Can you work these out from the model? Positions are in its coordinate system, mm. Face numbers are marked on the shaded views. A direction names the side the tool comes from. Give positions to 0.01 mm unless a question says otherwise; leave off trailing zeros. Order: outer loops, then holes, each group sorted by start corner. A loop starts at its lowest first (then second) coordinate and runs counter-clockwise, first axis right, second up. Notation, with made-up numbers: (-4, 80.5) - (47, 80.5) arc R7 ccw to (47, 88.5) - close; hole circle Ø4 at (15, -8). An arc over 180 degrees is marked (long way). Use one line per item in the form item = value. Start each with the question number.
1) For pin 1 (6 mm diameter, centred on x = -25, z = -1.5, fed in from -Y); pin 2 (3 mm diameter, centred on x = -4, y = 9, fed in from +Z); pin 3 (0.8 mm diameter, centred on x = -11, y = 8, fed in from +Z); pin 4 (8 mm diameter, centred on x = -32, y = 8.5, fed in from -Z), each with a flat end and sliding along its axis, tell me the tip position at first contact or that it passes through.
2) Please list where these lines run through material, in increasing order: probe 1 along Y at (x, z) = (-31, -3); probe 2 along X at (y, z) = (-2.75, -16); probe 3 along Y at (x, z) = (20, -6.75).
3) We'd pull the mould along X, two halves only. Please class the marked faces 1, 2 and 3: released by +X, released by -X, zero draft, split by the parting line, or undercut.
4) Suppose I cut it at D-D, the plane x = 27. Write out the boundary of the cut face in (y, z), and give its area (3 significant figures).
5) Suppose I cut it at B-B, the plane z = -1.25. Write out the boundary of the cut face in (x, y) (3 decimals), and give its area (3 significant figures).
6) Suppose I cut it at C-C, the plane x = 7.5. Write out the boundary of the cut face in (y, z).
7) Suppose I cut it at A-A, the plane y = -1.5. Write out the boundary of the cut face in (x, z) (1 decimal).
8) Which directions (+Z, -Z, +X, -X, +Y, -Y) give clear straight access to the entire face, cutting with the end or side of a thin tool? Please do the marked faces 4, 5 and 6.
Autodesk Inventor part; units mm, degrees
ref_plane "YZ Plane" through (0, 0, 0) normal (1, 0, 0) x (0, 1, 0)
ref_plane "XZ Plane" through (0, 0, 0) normal (0, 1, 0) x (-1, 0, 0)
ref_plane "XY Plane" through (0, 0, 0) normal (0, 0, 1) x (1, 0, 0)
sketch "Sketch1" plane through (0, 0, 0) normal (0, 0, 1) x (1, 0, 0)
  line L0 (0, 12.3444) -> (0, -2.0574)
  line L1 (-35.56, 0) -> (35.56, 0)
  line L2 (-35.56, 0) -> (35.56, 0)
  line L3 (0, -2.0574) -> (0, 12.3444)
  line L4 (-12.319, 8.2169) -> (15.113, 8.2169)
  line L5 (-10.2108, 8.2169) -> (13.0048, 8.2169)
  circle A0 centre (-11.2649, 8.2169) radius 1.0541
  circle A1 centre (14.0589, 8.2169) radius 1.0541
  line L6 (-25.4, 10.287) -> (-25.4, 0)
  line L7 (-25.4, 0) -> (25.4, 0)
  line L8 (-25.4, 10.287) -> (25.4, 10.287)
  line L9 (25.4, 10.287) -> (25.4, 0)
  line L10 (25.4, 10.287) -> (14.0589, 10.287)
  line L11 (14.0589, 10.287) -> (14.0589, 7.1628)
  line L12 (14.0589, 9.271) -> (14.0589, 10.287)
  line L13 (14.0589, 8.2169) -> (15.113, 8.2169)
  circle A2 centre (-11.2649, 8.2169) radius 0.8001
  circle A3 centre (14.0589, 8.2169) radius 0.8001
  point P0 (0, 0)
  dimension "d0" = 27.432
  dimension "d1" = 23.2156
  dimension "d2" = 2.1082
  dimension "d3" = 10.287
  dimension "d4" = 50.8
  dimension "d5" = 11.3411
  dimension "d6" = 1.016
  dimension "d7" = 11.3411
  dimension "d8" = 0.254
  dimension "d9" = 0.254
extrude "Extrusion1" add sketch "Sketch1" against normal blind 5.08 contours L8 L11 A1 L4 L0 | L0 L1 L6 L8 | L4 A1 L11 L8 L9 L1 L0
extrude "Extrusion2" add sketch "Sketch1" against normal blind 5.08 contours A0 L4 A2 | L4 A2 A0 | A1 L11 A3 L4 | L4 A3 L11 A1 | A1 L4 A3 L11 | A2 L4 | L4 A2 | A3 L11 L4 | L4 L11 A3 | L11 A3 L4 A1 | A3 L4 L11 | L4 A3 L11
extrude "Extrusion3" add sketch "Sketch1" along normal blind 2.032 contours A2 L4 | L4 A2 | A3 L11 L4 | L4 L11 A3 | A3 L4 L11 | L4 A3 L11
sketch "Sketch2" plane through (-25.4, 0, 0) normal (0, -1, 0) x (1, 0, 0)
  line L0 (50.8, 0) -> (50.8, -5.08)
  line L1 (0, 0) -> (50.8, 0)
  line L2 (0, 0) -> (0, -5.08)
  line L3 (38.1, -5.08) -> (12.7, -5.08)
  line L4 (12.7, -17.78) -> (38.1, -17.78)
  arc A0 (38.1, -12.7) -> (38.1, -10.16) centre (38.1, -11.43) ccw
  arc A1 (12.7, -10.16) -> (12.7, -12.7) centre (12.7, -11.43) ccw
  line L5 (38.1, -17.78) -> (38.1, -12.7)
  line L6 (38.1, -10.16) -> (38.1, -5.08)
  line L7 (12.7, -5.08) -> (12.7, -10.16)
  line L8 (12.7, -12.7) -> (12.7, -17.78)
  line L9 (50.8, 0) -> (0, 0)
  line L10 (25.4, 0) -> (25.4, -33.3128)
  line L11 (25.4, -5.08) -> (25.4, -17.78)
  line L12 (50.8, -5.08) -> (0, -5.08)
  line L13 (50.8, -5.08) -> (0, -5.08)
  line L14 (50.8, -5.08) -> (42.0012, -20.32)
  line L15 (50.8, -5.08) -> (70.0547, -5.08) construction
  line L16 (0, -5.08) -> (8.7988, -20.32)
  line L17 (0, -5.08) -> (24.702, -5.08) construction
  line L18 (42.0012, -20.32) -> (8.7988, -20.32)
  dimension "d16" = 25.4
  dimension "d17" = 12.7
  dimension "d18" = 2.54
  dimension "d19" = 2.54
  dimension "d20" = 5.08
  dimension "d21" = 5.08
  dimension "d23" = 6.35
  dimension "d24" = 6.35
  dimension "d26" = 120
  dimension "d27" = 60
  dimension "d29" = 12.7
  dimension "d30" = 33.2024
  dimension "d31" = 19.2547
  dimension "d32" = 28.2328
  dimension "d33" = 26.098
extrude "Extrusion4" add sketch "Sketch2" against normal blind 10.287 contours L14 L18 L10 L4 L5 A0 L6 L12 | L6 A0 L5 L4 L10 L3 | L10 L4 L8 A1 L7 L3 | L18 L16 L12 L7 A1 L8 L4 L10
extrude "Extrusion5" add sketch "Sketch2" along normal blind 3.81 contours L6 A0 L5 L4 L10 L3 | L10 L4 L8 A1 L7 L3
sketch "Sketch4" plane through (-25.4, 0, 0) normal (0, -1, 0) x (1, 0, 0)
  line L0 (38.1, -5.08) -> (12.7, -5.08)
  line L1 (0, 0) -> (50.8, 0)
  line L2 (0, 0) -> (0, -5.08)
  line L3 (50.8, 0) -> (50.8, -5.08)
  line L4 (-15.875, -5.08) -> (66.675, -5.08)
  line L5 (25.4, 0) -> (25.4, -41.8957)
  line L6 (-15.875, 0) -> (-15.875, -5.08)
  line L7 (0, 0) -> (0, -5.08)
  line L8 (0, 0) -> (-15.875, 0)
  line L9 (0, 0) -> (0, -5.08)
  line L10 (50.8, 0) -> (0, 0)
  line L11 (50.8, 0) -> (50.8, -5.08)
  line L12 (50.8, 0) -> (66.675, 0)
  line L13 (66.675, 0) -> (66.675, -5.08)
  line L14 (-15.875, 0) -> (-15.875, 3.175)
  line L15 (-7.9375, 3.175) -> (-15.875, 3.175)
  line L16 (-7.9375, 3.175) -> (-7.9375, 0)
  line L17 (-15.875, -5.08) -> (-15.875, 3.175)
  line L18 (-15.875, 3.175) -> (-7.9375, 3.175)
  line L19 (-7.9375, 3.175) -> (-7.9375, 0)
  line L20 (50.8, 0) -> (0, 0)
  line L21 (-15.875, 0) -> (0, 0)
  line L22 (0, 0) -> (0, -5.08)
  line L23 (0, 0) -> (0, -5.08)
  line L24 (0, -5.08) -> (0, 0)
  line L25 (-15.875, -5.08) -> (66.675, -5.08)
  line L26 (25.4, 0) -> (25.4, -5.08)
  line L27 (12.7, -5.08) -> (38.1, -5.08)
  line L28 (66.675, 0) -> (66.675, -5.08)
  line L29 (66.675, 0) -> (66.675, 3.175)
  line L30 (58.7375, 3.175) -> (66.675, 3.175)
  line L31 (58.7375, 3.175) -> (58.7375, 0)
  line L32 (50.8, 0) -> (50.8, -5.08)
  line L33 (50.8, 0) -> (50.8, -5.08)
  line L34 (50.8, 0) -> (66.675, 0)
  line L35 (50.8, 0) -> (50.8, -5.08)
  line L36 (50.8, 0) -> (0, 0)
  line L37 (0, 0) -> (50.8, 0)
  line L38 (66.675, -5.08) -> (-15.875, -5.08)
  line L39 (66.675, -5.08) -> (66.675, 3.175)
  line L40 (66.675, 3.175) -> (58.7375, 3.175)
  line L41 (58.7375, 3.175) -> (58.7375, 0)
  line L42 (0, 0) -> (50.8, 0)
  line L43 (66.675, 0) -> (50.8, 0)
  line L44 (50.8, 0) -> (50.8, -5.08)
  line L45 (50.8, 0) -> (50.8, -5.08)
  line L46 (50.8, -5.08) -> (50.8, 0)
  line L47 (66.675, -5.08) -> (-15.875, -5.08)
  line L48 (-15.875, 0) -> (-7.9375, 0)
  dimension "d40" = 82.55
  dimension "d41" = 3.175
extrude "Extrusion6" add sketch "Sketch4" against normal blind 3.81 contours L0 L5 L1 L3 L4 | L0 L4 L2 L1 L5 | L3 L12 L13 L4 | L4 L6 L8 L2
extrude "Extrusion7" add sketch "Sketch4" along normal mid plane 7.62 contours L31 L30 L29 L12 | L8 L14 L15 L16
properties part number "LED_Holder_V1"
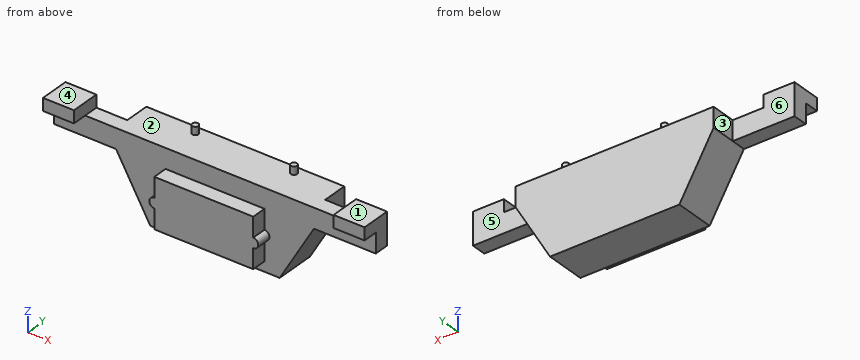
Result sheet:
q1.pin_1 = 0
q1.pin_2 = 0
q1.pin_3 = 2.03
q1.pin_4 = through
q2.probe_1 = 0 to 3.81
q2.probe_2 = -12.7 to 12.7
q2.probe_3 = 0 to 10.29
q3.face_1 = zero draft
q3.face_2 = undercut
q3.face_3 = released by -X
q4.outline = (0, -5.08) - (3.81, -5.08) - (3.81, 0) - (0, 0) - close
q4.area = 19.4 mm²
q5.outline = (-41.275, 0) - (41.275, 0) - (41.275, 3.81) - (25.4, 3.81) - (25.4, 10.287) - (-25.4, 10.287) - (-25.4, 3.81) - (-41.275, 3.81) - close
q5.area = 644 mm²
q6.outline = (-3.81, -17.78) - (0, -17.78) - (0, -20.32) - (10.29, -20.32) - (10.29, 0) - (0, 0) - (0, -5.08) - (-3.81, -5.08) - close
q7.outline = (-41.3, 0) - (-33.3, 0) - (-33.3, 3.2) - (-41.3, 3.2) - close; (-12.7, -17.8) - (12.7, -17.8) - (12.7, -12.7) arc R1.3 ccw to (12.7, -10.2) - (12.7, -5.1) - (-12.7, -5.1) - (-12.7, -10.2) arc R1.3 ccw to (-12.7, -12.7) - close; (33.3, 0) - (41.3, 0) - (41.3, 3.2) - (33.3, 3.2) - close
q8.face_4 = +Z, +X, -X, +Y, -Y
q8.face_5 = +Z, -Z, +X, +Y
q8.face_6 = +Z, -Z, -X, +Y
